Autodesk Inventor part; units mm, degrees
ref_plane "YZ Plane" through (0, 0, 0) normal (1, 0, 0) x (0, 1, 0)
ref_plane "XZ Plane" through (0, 0, 0) normal (0, 1, 0) x (-1, 0, 0)
ref_plane "XY Plane" through (0, 0, 0) normal (0, 0, 1) x (1, 0, 0)
sketch "Sketch1" plane through (0, 0, 0) normal (0, 1, 0) x (-1, 0, 0)
  line L0 (127.8549, 19.7947) -> (147.8549, 19.7947)
  line L1 (147.8549, 19.7947) -> (147.8549, 269.7947)
  line L2 (127.8549, 269.7947) -> (127.8549, 19.7947) construction
  line L3 (127.8549, 19.7947) -> (77.8549, 19.7947)
  line L4 (135.3134, 269.3194) -> (137.8549, 19.7947) construction
  circle A0 centre (136.5841, 144.5571) radius 2.65
  line L5 (136.5841, 144.5571) -> (137.8549, 19.7947) construction
  circle A1 centre (137.2195, 82.1759) radius 2.65
  line L6 (136.5841, 144.5571) -> (134.9234, 307.6106) construction
  line L7 (136.5841, 144.5571) -> (135.3134, 269.3194) construction
  circle A2 centre (135.9488, 206.9383) radius 2.65
  line L8 (110.2049, 216.8269) -> (110.2049, 41.8269) construction
  line L9 (110.2049, 216.8269) -> (121.6955, 226.4688) construction
  circle A3 centre (121.6955, 226.4688) radius 2.65
  circle A4 centre (110.2049, 216.8269) radius 2.65
  line L10 (92.3408, 41.8269) -> (92.3408, 61.8269) construction
  arc A5 (92.3408, 41.8269) -> (110.2049, 41.8269) centre (101.2728, 41.8269) ccw construction
  circle A6 centre (110.2049, 41.8269) radius 2.65
  circle A7 centre (92.3408, 61.8269) radius 2.65
  circle A8 centre (92.3408, 41.8269) radius 2.65
  line L11 (121.6955, 226.4688) -> (123.3989, 224.4387) construction
  line L12 (123.3989, 224.4387) -> (111.9082, 214.7969)
  line L13 (121.6955, 226.4688) -> (119.9921, 228.4988) construction
  line L14 (119.9921, 228.4988) -> (108.5015, 218.857)
  line L15 (110.2049, 216.8269) -> (107.5549, 216.8269) construction
  line L16 (107.5549, 216.8269) -> (107.5549, 41.8269)
  line L17 (112.8549, 41.8269) -> (112.8549, 216.8269)
  line L18 (94.9908, 61.8269) -> (94.9908, 41.8269)
  line L19 (89.6908, 61.8269) -> (89.6908, 41.8269)
  arc A9 (94.9908, 41.8269) -> (107.5549, 41.8269) centre (101.2728, 41.8269) ccw
  arc A10 (89.6908, 41.8269) -> (112.8549, 41.8269) centre (101.2728, 41.8269) ccw
  line L20 (92.3408, 61.8269) -> (94.9908, 61.8269) construction
  line L21 (77.8549, 19.7947) -> (77.8549, 191.4117)
  line L22 (112.8549, 129.3269) -> (127.8549, 129.3269) construction
  line L23 (127.8549, 241.4117) -> (147.8549, 241.4117)
  arc A11 (127.8549, 241.4117) -> (77.8549, 191.4117) centre (127.8549, 191.4117) ccw
  point P0 (0, 0)
  point P1 (112.8549, 215.5912)
  point P2 (89.6908, 41.8269)
  point P3 (77.8549, 241.4117)
  dimension "d0" = 20
  dimension "d1" = 250
  dimension "d11" = 5.3
  dimension "d12" = 5.3
  dimension "d13" = 5.3
  dimension "d16" = 175
  dimension "d17" = 15
  dimension "d18" = 130
  dimension "d19" = 5.3
  dimension "d20" = 5.3
  dimension "d21" = 20
  dimension "d22" = 5.3
  dimension "d23" = 5.3
  dimension "d24" = 5.3
  dimension "d25" = 50
  dimension "d26" = 15
  dimension "d29" = 10
  dimension "d30" = 10
  dimension "d31" = 50
extrude "Extrusion1" add sketch "Sketch1" against normal blind 10
properties part number "slothinge"
Work out the finished part from the listing and answer in its coordinate system (mm). A direction names the side the tool comes from. Round coordinates to 2 decimals unless told otherwise and drop trailing zeros. Write each loop counter-clockwise with the first axis right and the second up, starting at its lowest first coordinate (ties: lowest second). Pieces come first, ordered by that corner, then holes. Notation, with made-up numbers: (-14, 39) -> (1, 39) arc R25 ccw to (1, 68) -> close; hole circle Ø10 at (-3, 29). An arc over 180 degrees is marked (long way). Write each question's results on one line, items separated by ' | '.
1) For a pull along X with two mould halves and no side action, classify faces 1 (the flat face through (-120, 0, 132)), 2 (the cylindrical face through (-136.875, -4.93, 84.803)), 3 (the flat face through (-147.855, -5, 129)) as +X half, -X half, draft (parallel to the pull), parting line (faces both ways), or undercut.
Findings:
face 1: draft | face 2: undercut | face 3: -X half
2) The part is cut by section A-A (z = 89). Write down the section's boundary in (x, y), and give its area (3 significant figures).
Findings:
outline: (-147.85, -10) -> (-112.85, -10) -> (-112.85, 0) -> (-147.85, 0) -> close; (-107.55, -10) -> (-77.85, -10) -> (-77.85, 0) -> (-107.55, 0) -> close | area: 647 mm²
3) Which of the six approach directions +Z, -Z, +X, -X, +Y, -Y give full straight-line access (tool end or side, diameter ignored) to faces 4 (the flat face through (-77.855, -5, 104)), 5 (the flat face through (-89.691, -5, 52))?
Findings:
face 4: +Z, -Z, +X, +Y, -Y | face 5: +Y, -Y
4) Consider line 1 along X through (y, z) = (-9.25, 59.5); line 2 along X through (y, z) = (-3.75, 86.5); line 3 along Z through (x, y) = (-137, -6.75) (3 decimals). Determine where each line is inside the solid, lowest interval first. Write a range as [from, to].
Findings:
line 1: x = [-147.85, -112.85], [-107.55, -94.99], [-89.69, -77.85] | line 2: x = [-147.85, -112.85], [-107.55, -77.85] | line 3: z = [19.795, 79.535], [84.817, 141.94], [147.174, 204.506], [209.371, 241.412]
5) The part is cut by section B-B (x = -92.5). Write down the section's boundary in (y, z).
Findings:
outline: (-10, 19.79) -> (0, 19.79) -> (0, 34.27) -> (-10, 34.27) -> close; (-10, 64.47) -> (0, 64.47) -> (0, 226.77) -> (-10, 226.77) -> close
6) The part is cut by section C-C (y = -1.75). Write down the section's boundary in (x, z).
Findings:
outline: (-147.85, 19.79) -> (-77.85, 19.79) -> (-77.85, 191.41) arc R50 ccw to (-127.85, 241.41) -> (-147.85, 241.41) -> close; hole circle Ø5.3 at (-137.22, 82.18); hole circle Ø5.3 at (-136.58, 144.56); hole circle Ø5.3 at (-135.95, 206.94); hole (-123.4, 224.44) -> (-112.85, 215.59) -> (-112.85, 41.83) arc R11.58 ccw to (-89.69, 41.83) -> (-89.69, 61.83) arc R2.65 ccw to (-94.99, 61.83) -> (-94.99, 41.83) arc R6.28 cw to (-107.55, 41.83) -> (-107.55, 216.83) arc R2.65 ccw to (-108.5, 218.86) -> (-119.99, 228.5) arc R2.65 ccw to start
7) Flat-ended cylindrical pins translate along their axes: pin 1 (1 mm diameter, centred on x = -110.5, y = -6.5, fed in from +Z); pin 2 (4 mm diameter, centred on y = -8.5, z = 219, fed in from +X). Find the tip coordinate at first contact, or state that the pin passes through.
Findings:
pin 1: stops at z = 238.49 | pin 2: stops at x = -84.9
